The model under review builds one solid part; all positions refer to its coordinate system, in mm. Face numbers are marked on the shaded views. Give positions to 0.01 mm unless a question says otherwise; leave off trailing zeros. Loops run counter-clockwise (first coordinate to the right, second up) from the corner with the lowest first, then second, coordinate; pieces in that order, holes last. Notation, with made-up numbers: M -20.5,37.25 L 25.5,37.25 A36 cw 25.5,72.25 Z; hole C 37.25,32.5 d3. An arc over 180 degrees is marked long. Put each result on its own line as item: value. Start each with the question number.
Autodesk Inventor part; units mm, degrees
ref_plane "YZ Plane" through (0, 0, 0) normal (1, 0, 0) x (0, 1, 0)
ref_plane "XZ Plane" through (0, 0, 0) normal (0, 1, 0) x (-1, 0, 0)
ref_plane "XY Plane" through (0, 0, 0) normal (0, 0, 1) x (1, 0, 0)
sketch "Sketch1" plane through (0, 0, 0) normal (1, 0, 0) x (0, 1, 0)
  line L0 (-65, 43) -> (65, 43)
  line L1 (65, 43) -> (65, -43)
  line L2 (65, -43) -> (-65, -43)
  line L3 (-65, -43) -> (-65, 43)
  line L4 (-65, 43) -> (65, -43) construction
  line L5 (65, 43) -> (-65, -43) construction
  point P0 (0, 0)
  dimension "d0" = 130
  dimension "d1" = 86
extrude "Extrusion1" add sketch "Sketch1" along normal blind 12
sketch "Sketch2" plane through (12, 0, 0) normal (1, 0, 0) x (0, 0, -1)
  circle A0 centre (-25, 49.2145) radius 3.25
  circle A1 centre (-25, -49.2145) radius 3.25
  line L0 (-43, 65) -> (-43, -65)
  line L1 (-25, 49.2145) -> (-25, -49.2145) construction
  line L2 (-43, 0) -> (-25, 0) construction
  circle A2 centre (24.2145, 0) radius 3.25
  line L3 (-25, 0) -> (24.2145, 0) construction
  circle A3 centre (-25, 0) radius 30.5
  point P0 (0, 0)
  dimension "d4" = 18
  dimension "d5" = 18
  dimension "d6" = 98.429
  dimension "d7" = 6.5
  dimension "d8" = 6.5
  dimension "d9" = 6.5
  dimension "d10" = 49.2145
  dimension "d13" = 61
extrude "Extrusion2" cut sketch "Sketch2" against normal through all
ref_plane "Work Plane1" through (6, 0, 0) normal (1, 0, 0) x (0, 0, -1)
sketch "Sketch3" plane through (0, 65, 43) normal (0, 0, 1) x (1, 0, 0)
  circle A0 centre (6, -8) radius 3 construction
  circle A1 centre (6, -104) radius 3
  line L0 (0, -130) -> (12, -130)
  line L1 (6, -130) -> (6, 0) construction
  line L2 (0, 0) -> (12, 0)
  circle A2 centre (6, -26) radius 3
  point P0 (0, -65)
  dimension "d14" = 6
  dimension "d15" = 26
  dimension "d17" = 8
  dimension "d29" = 18
extrude "Extrusion3" cut sketch "Sketch3" against normal blind 15
sketch "Sketch4" plane through (0, -65, -43) normal (0, -1, 0) x (1, 0, 0)
  circle A0 centre (6, 15) radius 3
  circle A1 centre (6, 59) radius 3
  line L0 (0, 0) -> (12, 0)
  line L1 (6, 0) -> (6, 86) construction
  line L2 (0, 86) -> (12, 86)
  point P0 (0, 43)
  dimension "d21" = 6
  dimension "d22" = 27
  dimension "d23" = 15
extrude "Extrusion4" cut sketch "Sketch4" against normal blind 15
sketch "Sketch6" plane through (0, 0, 0) normal (-1, 0, 0) x (0, 0, 1)
  circle A0 centre (-33, 35) radius 3 construction
  circle A1 centre (-13, 35) radius 3 construction
  circle A2 centre (-13, 35) radius 3.25
  circle A3 centre (-33, 35) radius 3.25
  point P0 (0, 0)
  dimension "d32" = 0.25
  dimension "d33" = 0.25
extrude "Extrusion6" cut sketch "Sketch6" against normal through all
thread "Thread1"
thread "Thread2"
thread "Thread3"
thread "Thread4"
equation "\"d10\" = 0.5 * d6"
properties part number "MotorHolderLongAxis"
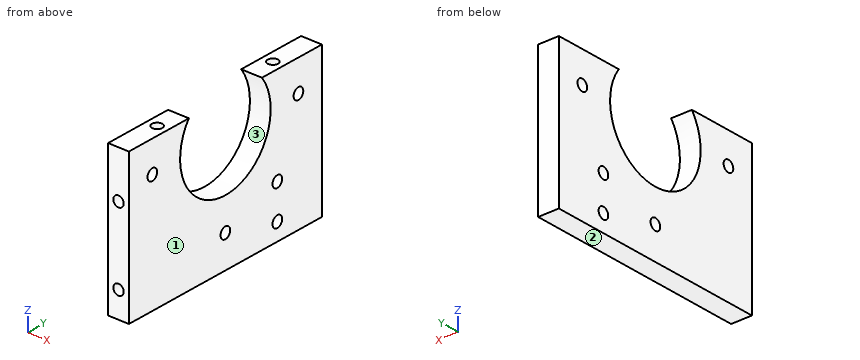
Item 1: Consider section C-C, the plane z = 7. Write out the cut boundary in (x, y).
Item 2: Consider section B-B, the plane y = 0. Write out the cut boundary in (x, z).
Item 3: Consider section D-D, the plane x = 6. Write out the cut boundary in (y, z), plus the area to 3 significant figures.
Item 4: Consider section A-A, the plane z = 25. Write out the cut boundary in (x, y), plus the area to 3 significant figures.
Item 5: Clearance check with flat-ended pins moving along their axes: pin 1 Ø1.8 at (x, z) = (6, -29) entering from -Y; pin 2 Ø3.5 at (x, y) = (6, -39) entering from +Z. State where each tip first meets the part, or that it passes through.
Item 6: To check wall thickness, follow L1, parallel to Z at x = 6, y = -61; L2, parallel to Y at x = 4.25, z = 25; L3, parallel to Y at x = 2.5, z = -33. State the ranges of each line that lie inside material, in increasing order. Write a range as [from, to].
Item 7: Draft analysis for pull direction Z (two halves, no side actions). For the marked faces 1, 2 and 3, state which applies: +Z half, -Z half, draft (parallel to the pull), parting line (faces both ways), or undercut.
Report:
1. outline: M 0,-65 L 12,-65 L 12,-24.62 L 0,-24.62 Z; M 0,24.62 L 12,24.62 L 12,65 L 0,65 Z
2. outline: M 0,-43 L 12,-43 L 12,-27.46 L 0,-27.46 Z; M 0,-20.96 L 12,-20.96 L 12,-5.5 L 0,-5.5 Z
3. outline: M -65,-43 L 65,-43 L 65,43 L 42,43 L 42,28 L 36,28 L 36,43 L 24.62,43 A30.5 cw long -24.62,43 L -36,43 L -36,28 L -42,28 L -42,43 L -65,43 L -65,19 L -50,19 L -50,13 L -65,13 L -65,-25 L -50,-25 L -50,-31 L -65,-31 Z; hole C -49.21,25 d6.5; hole C 0,-24.21 d6.5; hole C 35,-33 d6.5; hole C 35,-13 d6.5; hole C 49.21,25 d6.5
3. area: 8,160 mm²
4. outline: M 0,-65 L 12,-65 L 12,-52.46 L 0,-52.46 Z; M 0,-45.96 L 12,-45.96 L 12,-30.5 L 0,-30.5 Z; M 0,30.5 L 12,30.5 L 12,45.96 L 0,45.96 Z; M 0,52.46 L 12,52.46 L 12,65 L 0,65 Z
4. area: 672 mm²
5. pin 1: y = -50
5. pin 2: z = 28
6. L1: [-43, -31], [-25, 13], [19, 43]
6. L2: [-65, -52.46], [-45.96, -30.5], [30.5, 45.96], [52.46, 65]
6. L3: [-65, 31.75], [38.25, 65]
7. face 1: draft
7. face 2: -Z half
7. face 3: undercut
